Input: part model. Units: mm. Frame: model coordinates. A direction names the side the tool comes from. Coordinates: 2 decimals unless noted, no trailing zeros. Order: outer loops, then holes, each group sorted by start corner. A loop starts at its lowest first (then second) coordinate and runs counter-clockwise, first axis right, second up. Notation, with made-up numbers: M -32,62 L 4,62 A23 cw 4,89 Z; hole C 68.5,43 d3. An arc over 180 degrees is marked long. Answer in a Markdown table with one row per item.
from build123d import *

# Parameters (mm, degrees)
BOSS_EXTRUDE1_DEPTH = 3.9
SKETCH2_W           = 0.125
SKETCH2_H           = 0.1
CUT_EXTRUDE1_DEPTH  = 11.306581635
FILLET1_R           = 1
FILLET2_R           = 1.125
SKETCH3_W           = 2.65
SKETCH3_H           = 1.1
CUT_EXTRUDE2_DEPTH  = 8.91426718
SKETCH4_R           = 1.55
CUT_EXTRUDE3_DEPTH  = 8.91426718


with BuildPart() as part:
    # Sketch1 → Boss-Extrude1 (new, symmetric)
    with BuildSketch(Plane(origin=(0, 0, 0), x_dir=(0, 0, -1), z_dir=(1, 0, 0))):
        with BuildLine():
            Line((-5.125, -3.5), (-5.125, -1.1))
            ThreePointArc((-5.125, -1.1), (-4.802817459, -0.322182541), (-4.025, 0))
            Line((-4.025, 0), (-3.75, 0))
            Line((-3.75, 0), (-3.75, 0.1))
            Line((-3.75, 0.1), (-3.875, 0.1))
            Line((-3.875, 0.1), (-3.875, 1.1))
            Line((-3.875, 1.1), (3.875, 1.1))
            Line((3.875, 1.1), (3.875, 0.1))
            Line((3.875, 0.1), (3.75, 0.1))
            Line((3.75, 0.1), (3.75, 0))
            Line((3.75, 0), (4.025, 0))
            ThreePointArc((4.025, 0), (4.802817459, -0.322182541), (5.125, -1.1))
            Line((5.125, -1.1), (5.125, -3.5))
            Line((5.125, -3.5), (4.125, -3.5))
            Line((4.125, -3.5), (4.125, -1.1))
            ThreePointArc((4.125, -1.1), (4.095710678, -1.029289322), (4.025, -1))
            Line((4.025, -1), (-4.025, -1))
            ThreePointArc((-4.025, -1), (-4.095710678, -1.029289322), (-4.125, -1.1))
            Line((-4.125, -1.1), (-4.125, -3.5))
            Line((-4.125, -3.5), (-5.125, -3.5))
        make_face()
    extrude(amount=BOSS_EXTRUDE1_DEPTH, both=True)

    # Sketch2 → Cut-Extrude1 (cut, through all)
    with BuildSketch(Plane.XY.offset(3.75)):
        with Locations((3.8375, 0.05)):
            Rectangle(SKETCH2_W, SKETCH2_H)
        with Locations((-3.8375, 0.05)):
            Rectangle(SKETCH2_W, SKETCH2_H)
    extrude(amount=-CUT_EXTRUDE1_DEPTH, mode=Mode.SUBTRACT)

    # Fillet1
    fillet1_edges = [part.edges().sort_by_distance(p)[0] for p in [
        (3.775, 0.05, -3.75),
        (3.775, 0.05, 3.75),
        (-3.775, 0.05, -3.75),
        (-3.775, 0.05, 3.75),
    ]]
    fillet(fillet1_edges, radius=FILLET1_R)

    # Fillet2
    fillet2_edges = [part.edges().sort_by_distance(p)[0] for p in [
        (-3.9, 0.6, 3.875),
        (-3.9, 0.6, -3.875),
        (3.9, 0.6, -3.875),
        (3.9, 0.6, 3.875),
    ]]
    fillet(fillet2_edges, radius=FILLET2_R)

    # Sketch3 → Cut-Extrude2 (cut, through all)
    with BuildSketch(Plane.XZ.offset(3.5)):
        with Locations((2.575, 4.575)):
            Rectangle(SKETCH3_W, SKETCH3_H)
        with Locations((-2.575, 4.575)):
            Rectangle(SKETCH3_W, SKETCH3_H)
    cut_extrude2 = extrude(amount=-CUT_EXTRUDE2_DEPTH, mode=Mode.SUBTRACT)

    # Mirror1: Cut-Extrude2 across plane
    add(cut_extrude2.mirror(Plane.XY), mode=Mode.SUBTRACT)

    # Sketch4 → Cut-Extrude3 (cut, through all)
    with BuildSketch(Plane(origin=(0, 1.1, 0), x_dir=(1, 0, 0), z_dir=(0, 1, 0))):
        with Locations(Location((0, 0, 0), (0, 0, 270))):
            Circle(SKETCH4_R)
    extrude(amount=-CUT_EXTRUDE3_DEPTH, mode=Mode.SUBTRACT)


solid = part.part
1) Mould query, pull axis Y, two halves, no side actions, for faces 6 (the face through (0, -3.5, 4.6)), 7 (the face through (0.02, -0.33, 4.81)), 8 (the face through (3.579, 0.607, 3.537)). Classes: +Y half, -Y half, draft (parallel to the pull), parting line (faces both ways), or undercut.
Resolved:
| item | result |
|---|---|
| face 6 | -Y half |
| face 7 | +Y half |
| face 8 | draft |
2) Cut plane C-C, the plane x = 0. Output: boundary loops of the cut face in (y, z) (3 decimals).
Resolved:
| item | result |
|---|---|
| outline | M -3.5,-5.125 L -1.1,-5.125 A1.1 ccw 0,-4.025 L 0,-3.75 L 0.1,-3.75 L 0.1,-3.875 L 1.1,-3.875 L 1.1,-1.55 L -1,-1.55 L -1,-4.025 A0.1 cw -1.1,-4.125 L -3.5,-4.125 Z; M -3.5,4.125 L -1.1,4.125 A0.1 cw -1,4.025 L -1,1.55 L 1.1,1.55 L 1.1,3.875 L 0.1,3.875 L 0.1,3.75 L 0,3.75 L 0,4.025 A1.1 ccw -1.1,5.125 L -3.5,5.125 Z |
3) Cut plane A-A, the plane y = 0.25. Output: boundary loops of the cut face in (x, z) (3 decimals).
Resolved:
| item | result |
|---|---|
| outline | M -3.9,-2.75 A1.125 ccw -2.775,-3.875 L 2.775,-3.875 A1.125 ccw 3.9,-2.75 L 3.9,2.75 A1.125 ccw 2.775,3.875 L -2.775,3.875 A1.125 ccw -3.9,2.75 Z; hole C 0,0 d3.1 |
4) Cut plane B-B, the plane z = 0. Output: boundary loops of the cut face in (x, y) (3 decimals), and give its area (4 significant figures).
Resolved:
| item | result |
|---|---|
| outline | M -3.9,-1 L -1.55,-1 L -1.55,1.1 L -3.9,1.1 L -3.9,0.1 L -3.775,0.1 L -3.775,0 L -3.9,0 Z; M 1.55,-1 L 3.9,-1 L 3.9,0 L 3.775,0 L 3.775,0.1 L 3.9,0.1 L 3.9,1.1 L 1.55,1.1 Z |
| area | 9.845 mm2 |
5) Reachability of faces 1 (the face through (1.25, -1.8, -4.6)), 2 (the face through (2, -1, 0)), 3 (the face through (0, 0.6, -3.875)), 4 (the face through (-1.25, -1.8, 4.6)), 5 (the face through (3.562, 0.593, -3.554)) from +Z, -Z, +X, -X, +Y, -Y: full face, straight path, thin tool, end or side. Return the list, or none.
Resolved:
| item | result |
|---|---|
| face 1 | -Z, +X, +Y, -Y |
| face 2 | +X, -X, -Y |
| face 3 | -Z, +X, -X, +Y |
| face 4 | +Z, -X, +Y, -Y |
| face 5 | -Z, +X, +Y |
6) Contact query for flat-ended pins moving along their axis: pin 1 (3.5 mm diameter, centred on x = 0, z = 0, fed in from +Y); pin 2 (0.8 mm diameter, centred on x = 2, y = -0.5, fed in from +Z) (3 decimals); pin 3 (0.8 mm diameter, centred on x = 0.5, y = 1, fed in from -Z) (3 decimals); pin 4 (1.2 mm diameter, centred on y = -2.5, z = -4.5, fed in from +X). Output: stop coordinate, or through.
Resolved:
| item | result |
|---|---|
| pin 1 | stops at y = 1.1 |
| pin 2 | stops at z = 4.025 |
| pin 3 | stops at z = -3.875 |
| pin 4 | stops at x = 1.25 |
7) Cut plane D-D, the plane y = -3. Output: boundary loops of the cut face in (x, z) (3 decimals), and give its area (3 significant figures).
Resolved:
| item | result |
|---|---|
| outline | M -1.25,-5.125 L 1.25,-5.125 L 1.25,-4.125 L -1.25,-4.125 Z; M -1.25,4.125 L 1.25,4.125 L 1.25,5.125 L -1.25,5.125 Z |
| area | 5.00 mm2 |
8) Material intervals for probe 1 along X at (y, z) = (-0.1, 0); probe 2 along Y at (x, z) = (-0.25, -2.5); probe 3 along Z at (x, y) = (-0.5, -0.8), sorted ascending.
Resolved:
| item | result |
|---|---|
| probe 1 | x = -3.9 to -1.55, 1.55 to 3.9 |
| probe 2 | y = -1 to 1.1 |
| probe 3 | z = -5.08 to -1.47, 1.47 to 5.08 |
